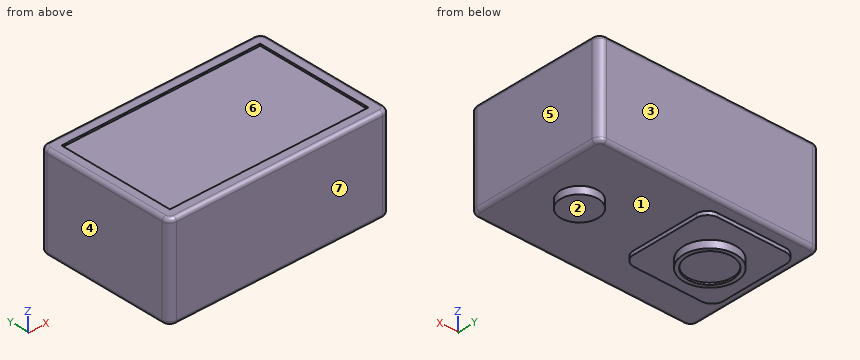
```python
from build123d import *

# Parameters (mm, degrees)
SKETCH1_W           = 59
SKETCH1_H           = 37
BOSS_EXTRUDE1_DEPTH = 12.5
SKETCH2_R           = 7
BOSS_EXTRUDE2_DEPTH = 3
FILLET1_R           = 2
BOSS_EXTRUDE3_DEPTH = 1
SKETCH4_R           = 6
CUT_EXTRUDE1_DEPTH  = 0.5
SKETCH5_R           = 5
BOSS_EXTRUDE4_DEPTH = 2
FILLET2_R           = 1
SKETCH6_W           = 53
SKETCH6_H           = 31
CUT_EXTRUDE2_DEPTH  = 0.5


with BuildPart() as part:
    # Sketch1 → Boss-Extrude1 (new, symmetric)
    with BuildSketch(Plane.XY):
        with Locations((0, 63.5)):
            Rectangle(SKETCH1_W, SKETCH1_H)
    extrude(amount=BOSS_EXTRUDE1_DEPTH, both=True)

    # Sketch2 → Boss-Extrude2 (add)
    with BuildSketch(Plane(origin=(0, 0, -12.5), x_dir=(-1, 0, 0), z_dir=(0, 0, -1))):
        with Locations(Location((14.5, 66.5, 0), (0, 0, 180))):
            Circle(SKETCH2_R)
    extrude(amount=BOSS_EXTRUDE2_DEPTH)

    # Fillet1
    fillet1_edges = [part.edges().sort_by_distance(p)[0] for p in [
        (-29.5, 82, 0),
        (29.5, 82, 0),
        (29.5, 45, 0),
        (-29.5, 45, 0),
    ]]
    fillet(fillet1_edges, radius=FILLET1_R)

    # Sketch3 → Boss-Extrude3 (add, symmetric)
    with BuildSketch(Plane(origin=(0, 0, -12.5), x_dir=(-1, 0, 0), z_dir=(0, 0, -1))):
        with BuildLine():
            Line((5.5, 78.5), (23.5, 78.5))
            ThreePointArc((23.5, 78.5), (25.621320344, 77.621320344), (26.5, 75.5))
            Line((26.5, 75.5), (26.5, 57.5))
            ThreePointArc((26.5, 57.5), (25.621320344, 55.378679656), (23.5, 54.5))
            Line((23.5, 54.5), (5.5, 54.5))
            ThreePointArc((5.5, 54.5), (3.378679656, 55.378679656), (2.5, 57.5))
            Line((2.5, 57.5), (2.5, 75.5))
            ThreePointArc((2.5, 75.5), (3.378679656, 77.621320344), (5.5, 78.5))
        make_face()
    extrude(amount=BOSS_EXTRUDE3_DEPTH, both=True)

    # Sketch4 → Cut-Extrude1 (cut)
    with BuildSketch(Plane(origin=(0, 0, -15.5), x_dir=(-1, 0, 0), z_dir=(0, 0, -1))):
        with Locations((14.5, 66.5)):
            Circle(SKETCH4_R)
    extrude(amount=-CUT_EXTRUDE1_DEPTH, mode=Mode.SUBTRACT)

    # Sketch5 → Boss-Extrude4 (add)
    with BuildSketch(Plane(origin=(0, 0, -12.5), x_dir=(-1, 0, 0), z_dir=(0, 0, -1))):
        with Locations(Location((-17.5, 63.5, 0), (0, 0, 180))):
            Circle(SKETCH5_R)
    extrude(amount=BOSS_EXTRUDE4_DEPTH)

    # Fillet2
    fillet2_edges = [part.edges().sort_by_distance(p)[0] for p in [
        (29.5, 63.5, -12.5),
        (29.5, 63.5, 12.5),
        (-29.5, 63.5, -12.5),
        (0, 82, -12.5),
        (0, 45, -12.5),
        (-28.914213562, 81.414213562, -12.5),
        (-28.914213562, 45.585786438, -12.5),
        (28.914213562, 81.414213562, -12.5),
        (28.914213562, 45.585786438, -12.5),
        (0, 45, 12.5),
        (-29.5, 63.5, 12.5),
        (0, 82, 12.5),
        (-28.914213562, 81.414213562, 12.5),
        (-28.914213562, 45.585786438, 12.5),
        (28.914213562, 81.414213562, 12.5),
        (28.914213562, 45.585786438, 12.5),
    ]]
    fillet(fillet2_edges, radius=FILLET2_R)

    # Sketch6 → Cut-Extrude2 (cut)
    with BuildSketch(Plane.XY.offset(12.5)):
        with Locations((0, 63.5)):
            Rectangle(SKETCH6_W, SKETCH6_H)
    extrude(amount=-CUT_EXTRUDE2_DEPTH, mode=Mode.SUBTRACT)


solid = part.part
```
The listing builds one solid part. Answer for the finished solid, in the listing's coordinates (mm). Face numbers are marked on the shaded views. A direction names the side the tool comes from. Coordinates: 2 decimals unless noted, no trailing zeros. Write each loop counter-clockwise with the first axis right and the second up, starting at its lowest first coordinate (ties: lowest second). Pieces come first, ordered by that corner, then holes. Notation, with made-up numbers: (-36.5, -29.5) - (-16.5, -29.5) arc R10 cw to (-16.5, -13.5) - close; hole circle Ø7 at (16.25, 15). An arc over 180 degrees is marked (long way). One line per item, written item: value.
1) Find section C-C (x = 17.5). Give the vertices of the cut face in (y, z).
Geometry check:
outline: (45, -11.5) arc R1 ccw to (46, -12.5) - (58.5, -12.5) - (58.5, -14.5) - (68.5, -14.5) - (68.5, -12.5) - (81, -12.5) arc R1 ccw to (82, -11.5) - (82, 11.5) arc R1 ccw to (81, 12.5) - (79, 12.5) - (79, 12) - (48, 12) - (48, 12.5) - (46, 12.5) arc R1 ccw to (45, 11.5) - close
2) A tool of negligible diameter and unlimited length cuts with its end or side. For the marked faces 1, 2 and 3, from which of +Z, -Z, +X, -X, +Y, -Y can it reach the whole face along a straight path? Write none if from no direction.
Geometry check:
face 1: -Z
face 2: -Z, +X, +Y, -Y
face 3: +Z, -Z, +X, -X, +Y
3) Consider line 1 along Y through (x, z) = (-14.5, -15.1); line 2 along Z through (x, y) = (2.5, 49.5); line 3 along Z through (x, y) = (-4.5, 55). Determine where each line is inside the solid, lowest interval first. Write a range as from..to.
Geometry check:
line 1: y = 59.5..60.5, 72.5..73.5
line 2: z = -12.5..12
line 3: z = -13.5..12
4) Find section D-D (y = 56). Give the vertices of the cut face in (x, z), and give its area (3 significant figures).
Geometry check:
outline: (-29.5, -11.5) arc R1 ccw to (-28.5, -12.5) - (-26.1, -12.5) - (-26.1, -13.5) - (-2.9, -13.5) - (-2.9, -12.5) - (28.5, -12.5) arc R1 ccw to (29.5, -11.5) - (29.5, 11.5) arc R1 ccw to (28.5, 12.5) - (26.5, 12.5) - (26.5, 12) - (-26.5, 12) - (-26.5, 12.5) - (-28.5, 12.5) arc R1 ccw to (-29.5, 11.5) - close
area: 1,470 mm2
5) Find section A-A (x = -14.5). Give the vertices of the cut face in (y, z).
Geometry check:
outline: (45, -11.5) arc R1 ccw to (46, -12.5) - (54.5, -12.5) - (54.5, -13.5) - (59.5, -13.5) - (59.5, -15.5) - (60.5, -15.5) - (60.5, -15) - (72.5, -15) - (72.5, -15.5) - (73.5, -15.5) - (73.5, -13.5) - (78.5, -13.5) - (78.5, -12.5) - (81, -12.5) arc R1 ccw to (82, -11.5) - (82, 11.5) arc R1 ccw to (81, 12.5) - (79, 12.5) - (79, 12) - (48, 12) - (48, 12.5) - (46, 12.5) arc R1 ccw to (45, 11.5) - close
6) Each of these flat-tipped pins is pushed along its axis until it touches: pin 1 Ø12 at (x, y) = (20.5, 50) entering from +Z; pin 2 Ø9.5 at (x, y) = (-14.5, 66.5) entering from -Z; pin 3 Ø0.8 at (x, z) = (-11.5, -13) entering from -Y; pin 4 Ø0.5 at (y, z) = (69.5, -13) entering from +X. Where does it stop, or does it pass through?
Geometry check:
pin 1: stops at z = 12.5
pin 2: stops at z = -15
pin 3: stops at y = 54.5
pin 4: stops at x = -2.5
7) For a pull along X with two mould halves and no side action, classify the marked faces 4, 5, 6 and 7 as pulls with the +X half, pulls with the -X half, needs draft (parallel to the pull), parting line crosses it, or undercut.
Geometry check:
face 4: pulls with the -X half
face 5: pulls with the +X half
face 6: undercut
face 7: needs draft
8) Find section B-B (y = 49.5). Give the vertices of the cut face in (x, z).
Geometry check:
outline: (-29.5, -11.5) arc R1 ccw to (-28.5, -12.5) - (28.5, -12.5) arc R1 ccw to (29.5, -11.5) - (29.5, 11.5) arc R1 ccw to (28.5, 12.5) - (26.5, 12.5) - (26.5, 12) - (-26.5, 12) - (-26.5, 12.5) - (-28.5, 12.5) arc R1 ccw to (-29.5, 11.5) - close
